```python
from build123d import *

# Parameters (mm, degrees)
SALIENTE_EXTRUIR1_DEPTH = 15
CROQUIS2_R              = 16.164040976
SALIENTE_EXTRUIR2_DEPTH = 25
CROQUIS3_R              = 17.134212929
SALIENTE_EXTRUIR3_DEPTH = 20
CROQUIS4_R              = 12.514075771
CORTAR_EXTRUIR1_DEPTH   = 61


with BuildPart() as part:
    # Croquis1 → Saliente-Extruir1 (new body)
    with BuildSketch(Plane(origin=(0, 0, 0), x_dir=(1, 0, 0), z_dir=(0, 1, 0))):
        Polygon((22.5, 0), (11.25, 19.485571585), (-11.25, 19.485571585), (-22.5, 0), (-11.25, -19.485571585), (11.25, -19.485571585), align=None)
    extrude(amount=SALIENTE_EXTRUIR1_DEPTH)

    # Croquis2 → Saliente-Extruir2 (add)
    with BuildSketch(Plane.XZ):
        Circle(CROQUIS2_R)
    extrude(amount=SALIENTE_EXTRUIR2_DEPTH)

    # Croquis3 → Saliente-Extruir3 (add)
    with BuildSketch(Plane.XZ.offset(25)):
        Circle(CROQUIS3_R)
    extrude(amount=SALIENTE_EXTRUIR3_DEPTH)

    # Croquis4 → Cortar-Extruir1 (cut, through all)
    with BuildSketch(Plane.XZ.offset(45)):
        Circle(CROQUIS4_R)
    extrude(amount=-CORTAR_EXTRUIR1_DEPTH, mode=Mode.SUBTRACT)


solid = part.part
```
Work out the finished part from the listing and answer in its coordinate system (mm). A direction names the side the tool comes from. Give positions to 0.01 mm unless a question says otherwise; leave off trailing zeros. Loops run counter-clockwise (first coordinate to the right, second up) from the corner with the lowest first, then second, coordinate; pieces in that order, holes last. Notation, with made-up numbers: (26, 80.5) -> (51, 80.5) arc R14 cw to (51, 91.5) -> close; hole circle Ø3 at (40.5, 34). An arc over 180 degrees is marked (long way). Use CSV: the item, a comma, the result in double quotes.
1. Straight lines are drawn through the part: line 1 (Z direction, x = -0.5, y = -11); line 2 (Z direction, x = 0, y = 1); line 3 (Y direction, x = 4, z = -16). For each, find the intervals that lie inside material, in ascending order.
Found:
line 1,"-16.16 to -12.5, 12.5 to 16.16"
line 2,"-19.49 to -12.51, 12.51 to 19.49"
line 3,"-45 to -25, 0 to 15"
2. The part is cut by section C-C (z = 14). Write down the section's boundary in (x, y).
Found:
outline,"(-14.42, 0) -> (-8.08, 0) -> (-8.08, -25) -> (-9.88, -25) -> (-9.88, -45) -> (9.88, -45) -> (9.88, -25) -> (8.08, -25) -> (8.08, 0) -> (14.42, 0) -> (14.42, 15) -> (-14.42, 15) -> close"
3. The part is cut by section D-D (x = -9.5). Write down the section's boundary in (y, z), then the cut area to 3 significant figures.
Found:
outline,"(-45, -14.26) -> (-25, -14.26) -> (-25, -13.08) -> (0, -13.08) -> (0, -19.49) -> (15, -19.49) -> (15, -8.15) -> (-45, -8.15) -> close; (-45, 8.15) -> (15, 8.15) -> (15, 19.49) -> (0, 19.49) -> (0, 13.08) -> (-25, 13.08) -> (-25, 14.26) -> (-45, 14.26) -> close"
area,"831 mm^2"
4. A tool of negligible diameter and unlimited length cuts with its end or side. For faces 5 (the cylindrical face through (15.418, -12.325, 4.855)), 6 (the flat face through (-16.796, 7.395, -9.879)), 7 (the cylindrical face through (16.34, -34.86, 5.15)), from which of +Z, -Z, +X, -X, +Y, -Y can it reach the whole face along a straight path? Write none if from no direction.
Found:
face 5,"none"
face 6,"-Z, -X, +Y, -Y"
face 7,"-Y"
5. The part is cut by section A-A (x = 0). Write down the section's boundary in (y, z).
Found:
outline,"(-45, -17.13) -> (-25, -17.13) -> (-25, -16.16) -> (0, -16.16) -> (0, -19.49) -> (15, -19.49) -> (15, -12.51) -> (-45, -12.51) -> close; (-45, 12.51) -> (15, 12.51) -> (15, 19.49) -> (0, 19.49) -> (0, 16.16) -> (-25, 16.16) -> (-25, 17.13) -> (-45, 17.13) -> close"
6. The mould has two halves that part along Y. Classify faces 1 (the flat face through (1, -45, -13)), 2 (the flat face through (-16.95, 7.4, 9.61)), 3 (the flat face through (10, 15, -9)), 4 (the flat face through (-10, -25, -13)): +Y half, -Y half, draft (parallel to the pull), parting line (faces both ways), or undercut.
Found:
face 1,"-Y half"
face 2,"draft"
face 3,"+Y half"
face 4,"undercut"
7. The part is cut by section B-B (y = 9.5). Write down the section's boundary in (x, z), then the cut area to 3 significant figures.
Found:
outline,"(-22.5, 0) -> (-11.25, -19.49) -> (11.25, -19.49) -> (22.5, 0) -> (11.25, 19.49) -> (-11.25, 19.49) -> close; hole circle Ø25.03 at (0, 0)"
area,"823 mm^2"
8. Flat-ended cylindrical pins translate along their axes: pin 1 Ø4 at (y, z) = (-8.5, -12) entering from +X; pin 2 Ø11.5 at (x, z) = (8.5, 4) entering from -Y; pin 3 Ø2 at (x, y) = (-4, -10) entering from +Z; pin 4 Ø8 at (x, z) = (15, -15) entering from -Y. Find the tip coordinate at first contact, or state that the pin passes through.
Found:
pin 1,"x = 12.7"
pin 2,"y = -45"
pin 3,"z = 15.88"
pin 4,"y = 0"
